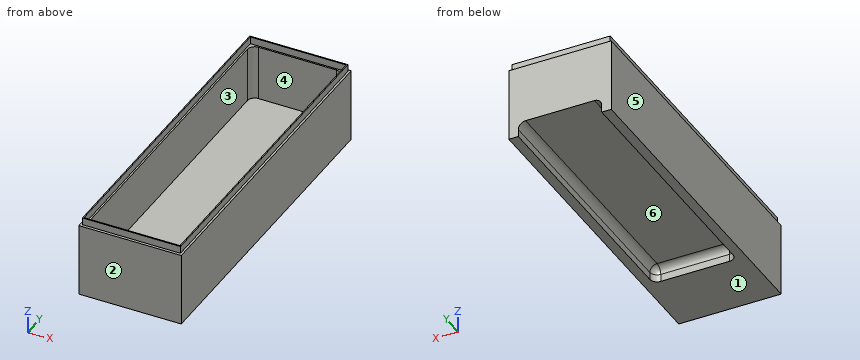
```python
from build123d import *

# Parameters (mm, degrees)
F0_W     = 70.739
F0_H     = 226.2886
F1_DEPTH = 50.8
F2_W     = 63.8302
F2_H     = 219.4306
F3_DEPTH = 38.1
F4_W     = 57.5818
F4_H     = 180.0606
F5_DEPTH = 10.16
F6_R     = 5
F7_W     = 67.691
F7_H     = 222.8596
F7_W_2   = 66.167
F7_H_2   = 221.3356
F8_DEPTH = 5


with BuildPart() as f1:
    # F0 (on Top) → F1 (new body)
    with BuildSketch(Plane.XY):
        with Locations((-8.073856, 34.662454)):
            Rectangle(F0_W, F0_H)
    extrude(amount=F1_DEPTH)

    # F2 (on face) → F3 (cut)
    with BuildSketch(Plane.XY.offset(50.8)):
        with Locations((-8.073856, 34.662454)):
            Rectangle(F2_W, F2_H)
    extrude(amount=-F3_DEPTH, mode=Mode.SUBTRACT)

    # F4 (on face) → F5 (cut)
    with BuildSketch(Plane(origin=(0, 0, 0), x_dir=(1, 0, 0), z_dir=(0, 0, -1))):
        with Locations((-8.073856, -57.776454)):
            Rectangle(F4_W, F4_H)
    extrude(amount=-F5_DEPTH, mode=Mode.SUBTRACT)

    # F6
    f6_edges = [f1.edges().sort_by_distance(p)[0] for p in [
        (-36.864756, 57.776454, 10.16),
        (20.717044, 57.776454, 10.16),
        (-8.073856, -32.253846, 10.16),
        (-36.864756, -32.253846, 5.08),
        (20.717044, -32.253846, 5.08),
        (-39.988956, -75.052846, 31.75),
        (-39.988956, 144.377754, 31.75),
        (23.841244, 144.377754, 31.75),
        (23.841244, -75.052846, 31.75),
    ]]
    fillet(f6_edges, radius=F6_R)

    # F7 (on face) → F8 (join)
    with BuildSketch(Plane.XY.offset(50.8)):
        with Locations((-8.073856, 34.852954)):
            Rectangle(F7_W, F7_H)
        with Locations((-8.073856, 34.852954)):
            Rectangle(F7_W_2, F7_H_2, mode=Mode.SUBTRACT)
    extrude(amount=F8_DEPTH)


solid = f1.part
```
CAD build for the part. Positions are in the model's coordinates, mm. Face numbers are marked on the shaded views. A direction names the side the tool comes from. Round coordinates to 2 decimals unless told otherwise and drop trailing zeros. Loops run counter-clockwise (first coordinate to the right, second up) from the corner with the lowest first, then second, coordinate; pieces in that order, holes last. Notation, with made-up numbers: M 19,-2 L 43,-2 A35 ccw 43,37 Z; hole C 75,62 d11. An arc over 180 degrees is marked long. Return JSON: item names as keys, results as strings. Group by question number.
(1) Saw through at A-A, the plane z = 23.5. List the corners of the cut face in (x, y), and give its area (3 significant figures).
(2) Drop flat-ended pins along their axis: P1, Ø4, axis at x = 2, y = 37, coming from the -Z side; P2, Ø4, axis at y = 7, z = 53, coming from the +X side; P3, Ø4, axis at x = -18, z = 2.5, coming from the +Y side. Give the stop position or say it passes through.
(3) Saw through at C-C, the plane x = -18. List the corners of the cut face in (y, z).
(4) Saw through at D-D, the plane y = -65. List the corners of the cut face in (x, z).
(5) Saw through at B-B, the plane y = 33. List the corners of the cut face in (x, z).
(6) Mould opens along Y. For the marked faces 1, 2 and 3 say: +Y half, -Y half, draft (parallel to the pull), parting line (faces both ways), or undercut.
(7) Tool access for the marked faces 4, 5 and 6: list every direction of +Z, -Z, +X, -X, +Y, -Y with a clear straight run to the whole face (end or side of a thin tool).
(8) Wall check: probe 1 along Y at (x, z) = (-14, 51); probe 2 along X at (y, z) = (2.5, 23.5); probe 3 along Y at (x, z) = (-16.5, 31.5). Give the ranges that are in metal, low to high. Write a range as [from, to].
Answer list:
{
 "1": {"outline": "M -43.44,-78.48 L 27.3,-78.48 L 27.3,147.81 L -43.44,147.81 Z; hole M -39.99,-70.05 A5 ccw -34.99,-75.05 L 18.84,-75.05 A5 ccw 23.84,-70.05 L 23.84,139.38 A5 ccw 18.84,144.38 L -34.99,144.38 A5 ccw -39.99,139.38 Z", "area": "2,020 mm2"},
 "2": {"P1": "z = 10.16", "P2": "x = 25.77", "P3": "y = -32.25"},
 "3": {"outline": "M -78.48,0 L -32.25,0 L -32.25,5.16 A5 cw -27.25,10.16 L 147.81,10.16 L 147.81,50.8 L 146.28,50.8 L 146.28,55.8 L 145.52,55.8 L 145.52,50.8 L 144.38,50.8 L 144.38,12.7 L -75.05,12.7 L -75.05,50.8 L -75.81,50.8 L -75.81,55.8 L -76.58,55.8 L -76.58,50.8 L -78.48,50.8 Z"},
 "4": {"outline": "M -43.44,0 L 27.3,0 L 27.3,50.8 L 25.77,50.8 L 25.77,55.8 L 25.01,55.8 L 25.01,50.8 L 23.84,50.8 L 23.84,12.7 L -39.99,12.7 L -39.99,50.8 L -41.16,50.8 L -41.16,55.8 L -41.92,55.8 L -41.92,50.8 L -43.44,50.8 Z"},
 "5": {"outline": "M -43.44,0 L -36.86,0 L -36.86,5.16 A5 cw -31.86,10.16 L 15.72,10.16 A5 cw 20.72,5.16 L 20.72,0 L 27.3,0 L 27.3,50.8 L 25.77,50.8 L 25.77,55.8 L 25.01,55.8 L 25.01,50.8 L 23.84,50.8 L 23.84,12.7 L -39.99,12.7 L -39.99,50.8 L -41.16,50.8 L -41.16,55.8 L -41.92,55.8 L -41.92,50.8 L -43.44,50.8 Z"},
 "6": {"face 1": "draft", "face 2": "-Y half", "face 3": "undercut"},
 "7": {"face 4": "+Z", "face 5": "+Z, -Z, -X, +Y, -Y", "face 6": "-Z, +Y"},
 "8": {"probe 1": "[-76.58, -75.81], [145.52, 146.28]", "probe 2": "[-43.44, -39.99], [23.84, 27.3]", "probe 3": "[-78.48, -75.05], [144.38, 147.81]"}
}
